Part model, mm, in its own coordinate system. A direction names the side the tool comes from. Coordinates: 2 decimals unless noted, no trailing zeros. Order: outer loops, then holes, each group sorted by start corner. A loop starts at its lowest first (then second) coordinate and runs counter-clockwise, first axis right, second up.
from build123d import *

# Parameters (mm, degrees)
BOSS_EXTRUDE1_DEPTH       = 17
SKETCH2_R                 = 3.05
CUT_EXTRUDE1_DEPTH        = 17
M3X0_5_TAPPED_HOLE1_D     = 2.5
M6X1_0_TAPPED_HOLE1_D     = 5
SKETCH7_R                 = 1
CUT_EXTRUDE2_DEPTH        = 5
M3X0_5_TAPPED_HOLE2_D     = 2.5
M3X0_5_TAPPED_HOLE2_DEPTH = 6
M3X0_5_TAPPED_HOLE2_TIP   = 0.751075774


with BuildPart() as part:
    # Sketch1 → Boss-Extrude1 (new body)
    with BuildSketch(Plane(origin=(0, 0, 0), x_dir=(1, 0, 0), z_dir=(0, 1, 0))):
        with BuildLine():
            Line((-7, 8), (7, 8))
            ThreePointArc((7, 8), (8.414213562, 7.414213562), (9, 6))
            Line((9, 6), (9, -6))
            ThreePointArc((9, -6), (8.414213562, -7.414213562), (7, -8))
            Line((7, -8), (-7, -8))
            ThreePointArc((-7, -8), (-8.414213562, -7.414213562), (-9, -6))
            Line((-9, -6), (-9, 6))
            ThreePointArc((-9, 6), (-8.414213562, 7.414213562), (-7, 8))
        make_face()
    extrude(amount=BOSS_EXTRUDE1_DEPTH)

    # Sketch2 → Cut-Extrude1 (cut, through all)
    with BuildSketch(Plane.XY.offset(8)):
        with Locations((3, 5)):
            Circle(SKETCH2_R)
    extrude(amount=-CUT_EXTRUDE1_DEPTH, mode=Mode.SUBTRACT)

    # M3x0.5 Tapped Hole1 (through all)
    with Locations(Plane.XY.offset(8)):
        with Locations((1, 12.5)):
            Hole(M3X0_5_TAPPED_HOLE1_D / 2)

    # M6x1.0 Tapped Hole1 (through all)
    with Locations(Plane(origin=(0, 17, 0), x_dir=(-1, 0, 0), z_dir=(0, 1, 0))):
        with Locations((4.5, 0)):
            Hole(M6X1_0_TAPPED_HOLE1_D / 2)

    # Sketch7 → Cut-Extrude2 (cut)
    with BuildSketch(Plane(origin=(0, 17, 0), x_dir=(1, 0, 0), z_dir=(0, 1, 0))):
        with Locations((-4.5, -8)):
            Circle(SKETCH7_R)
    extrude(amount=-CUT_EXTRUDE2_DEPTH, mode=Mode.SUBTRACT)

    # Sketch8 → Cut-Revolve1 (revolve, cut)
    with BuildSketch(Plane.ZY.offset(4.5), mode=Mode.PRIVATE) as cut_revolve1_sk:
        Polygon((4.796926452, 2.030181318), (5.9, 2.41), (9.273428811, 18.280734757), (8.29528121, 18.488646447), align=None)
    revolve(cut_revolve1_sk.sketch.rotate(Axis((-4.5, 1.132659385, 4.606152276), (0, 0.978147601, 0.207911691)), 180), axis=Axis((-4.5, 1.132659385, 4.606152276), (0, 0.978147601, 0.207911691)), mode=Mode.SUBTRACT)  # turned: the seam where the file's is

    # M3x0.5 Tapped Hole2
    with Locations(Plane(origin=(9, 0, 0), x_dir=(0, 0, -1), z_dir=(1, 0, 0))):
        with Locations((0, 5)):
            Hole(M3X0_5_TAPPED_HOLE2_D / 2, depth=M3X0_5_TAPPED_HOLE2_DEPTH)
            with Locations((0, 0, -(M3X0_5_TAPPED_HOLE2_DEPTH + M3X0_5_TAPPED_HOLE2_TIP / 2))):  # 118° drill point
                Cone(0, M3X0_5_TAPPED_HOLE2_D / 2, M3X0_5_TAPPED_HOLE2_TIP, mode=Mode.SUBTRACT)


solid = part.part
Q1. Cut at B-B on z = 0. Write the cut outline in (x, y).
Results list:
outline: (-9, 0) - (-7, 0) - (-7, 17) - (-9, 17) - close; (-2, 0) - (9, 0) - (9, 3.75) - (5.78, 3.75) arc R3.05 cw (long way) to (5.78, 6.25) - (9, 6.25) - (9, 17) - (-2, 17) - close; hole circle Ø2.5 at (1, 12.5)
Q2. Which spindle directions (+Z, -Z, +X, -X, +Y, -Y) get a long thin tool onto all of the face, cutting with end or side? Do faces 1 (the face through (7.37, 6.24, -0.16)), 2 (the face through (-4.672, 2.128, 4.841)), 3 (the face through (0, 8, 8)). Say none if no direction does.
Results list:
face 1: +X
face 2: none
face 3: +Z, +X, -X, +Y, -Y
Q3. Cut at A-A on x = 3. Write the cut outline in (y, z).
Results list:
outline: (0, -8) - (1.95, -8) - (1.95, 8) - (0, 8) - close; (8.05, -8) - (17, -8) - (17, 8) - (8.05, 8) - close
Q4. Cut at D-D on z = -4.25. Write the cut outline in (x, y).
Results list:
outline: (-9, 0) - (9, 0) - (9, 17) - (-9, 17) - close; hole circle Ø2.5 at (1, 12.5); hole circle Ø6.1 at (3, 5)
Q5. Mould opens along X. For faces 4 (the face through (-2.115, 8.381, 0.751)), 5 (the face through (0, 0, 0)), 6 (the face through (-8.43, 8.38, -7.4)) say: pulls with the +X half, pulls with the -X half, needs draft (parallel to the pull), parting line crosses it, or undercut.
Results list:
face 4: undercut
face 5: needs draft
face 6: pulls with the -X half
Q6. Pin check, flat tips, straight feed: pin 1 Ø1.5 at (x, z) = (5.5, 5) entering from -Y; pin 2 Ø1.5 at (y, z) = (5, 0) entering from +X. Stop position of each tip, or through.
Results list:
pin 1: stops at y = 0
pin 2: stops at x = 0.04
Q7. Cut at C-C on z = 2. Write the cut outline in (x, y), and give its area (3 significant figures).
Results list:
outline: (-9, 0) - (-6, 0) - (-6, 17) - (-9, 17) - close; (-3, 0) - (9, 0) - (9, 17) - (-3, 17) - close; hole circle Ø2.5 at (1, 12.5); hole circle Ø6.1 at (3, 5)
area: 221 mm2
Q8. Wall check: line 1 along Y through (x, z) = (8.3, 0); line 2 along Y through (x, z) = (3, -2); line 3 along X through (y, z) = (3, -1.75). Give the ranges that are in metal, low to high.
Results list:
line 1: y = 0 to 3.75, 6.25 to 17
line 2: y = 0 to 1.95, 8.05 to 17
line 3: x = -9 to -6.29, -2.71 to 0.7, 5.3 to 9
